Design review of the part built by this model. Coordinates are the model's own, in mm. Face numbers are marked on the shaded views. Round coordinates to 2 decimals unless told otherwise and drop trailing zeros. Loops run counter-clockwise (first coordinate to the right, second up) from the corner with the lowest first, then second, coordinate; pieces in that order, holes last. Notation, with made-up numbers: (27.25, 64.5) -> (86.25, 64.5) arc R14 ccw to (86.25, 85.5) -> close; hole circle Ø6 at (33, 36). An arc over 180 degrees is marked (long way). Use a Markdown table: item, result. Add a question column.
from build123d import *

# Parameters (mm, degrees)
F1_DEPTH = 30


with BuildPart() as f1:
    # F0 (on Front) → F1 (new body)
    with BuildSketch(Plane.XZ):
        with BuildLine():
            ThreePointArc((-2.471096, -22.384027), (-29.971096, 5.115973), (-57.471096, -22.384027))
            ThreePointArc((-57.471096, -22.384027), (-29.971096, -49.884027), (-2.471096, -22.384027))
        make_face()
        Polygon((-71.02997, 68.557098), (-104.971096, 34.615973), (-104.971096, -22.384027), (-104.971096, -97.384027), (123.028904, -97.384027), (123.028904, 34.615973), (11.060159, 68.557098), align=None)
        with BuildLine():
            ThreePointArc((-2.471096, -22.384027), (-29.971096, -49.884027), (-57.471096, -22.384027))
            ThreePointArc((-57.471096, -22.384027), (-29.971096, 5.115973), (-2.471096, -22.384027))
        make_face(mode=Mode.SUBTRACT)
    extrude(amount=F1_DEPTH)


solid = f1.part
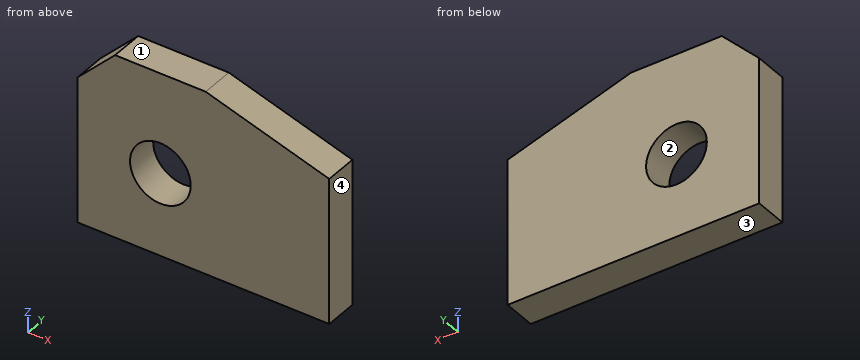
1. Consider section A-A on x = -42.5. State the section outline as (y, z) points, plus the area to 3 significant figures.
2. To check wall thickness, follow probe 1 along Z at (x, y) = (-30, -23.25); probe 2 along X at (y, z) = (-3.5, -10); probe 3 along X at (y, z) = (-18.75, -4). State the ranges of each line that lie inside material, in increasing order. Write a range as from..to.
3. Consider section C-C on y = -13.75. State the section outline as (x, z) points, plus the area to 3 significant figures.
4. Consider section D-D on x = 60.5. State the section outline as (y, z) points, plus the area to 3 significant figures.
5. Consider section B-B on z = -5.5. State the section outline as (x, y) points, plus the area to 3 significant figures.
6. Insertion check: P1, Ø1.5, axis at x = 99, y = -13.5, coming from the +Z side. The pin has a flat end and moves straight along its axis. Give the tip position at first contact, or say it passes through.
7. Mouldability with a two-part tool opening along Z and no side actions: class the marked faces 1, 2, 3 and 4 as +Z half, -Z half, draft (parallel to the pull), parting line (faces both ways), or undercut.
Verdict:
| question | item | result |
|---|---|---|
| 1 | outline | (-30, -97.38) -> (0, -97.38) -> (0, -46.86) -> (-30, -46.86) -> close; (-30, 2.1) -> (0, 2.1) -> (0, 68.56) -> (-30, 68.56) -> close |
| 1 | area | 3,510 mm² |
| 2 | probe 1 | z = -97.38..-49.88, 5.12..68.56 |
| 2 | probe 2 | x = -104.97..-54.52, -5.42..123.03 |
| 2 | probe 3 | x = -104.97..-50.42, -9.52..123.03 |
| 3 | outline | (-104.97, -97.38) -> (123.03, -97.38) -> (123.03, 34.62) -> (11.06, 68.56) -> (-71.03, 68.56) -> (-104.97, 34.62) -> close; hole circle Ø55 at (-29.97, -22.38) |
| 3 | area | 33,000 mm² |
| 4 | outline | (-30, -97.38) -> (0, -97.38) -> (0, 53.57) -> (-30, 53.57) -> close |
| 4 | area | 4,530 mm² |
| 5 | outline | (-104.97, -30) -> (-51.68, -30) -> (-51.68, 0) -> (-104.97, 0) -> close; (-8.26, -30) -> (123.03, -30) -> (123.03, 0) -> (-8.26, 0) -> close |
| 5 | area | 5,540 mm² |
| 6 | P1 | stops at z = 42.13 |
| 7 | face 1 | +Z half |
| 7 | face 2 | undercut |
| 7 | face 3 | -Z half |
| 7 | face 4 | draft |
